Input: part model. Units: mm. Frame: model coordinates. Face numbers are marked on the shaded views. A direction names the side the tool comes from. Coordinates: 2 decimals unless noted, no trailing zeros. Order: outer loops, then holes, each group sorted by start corner. A loop starts at its lowest first (then second) coordinate and runs counter-clockwise, first axis right, second up. Notation, with made-up numbers: (-12, 88.25) - (3, 88.25) arc R26 cw to (3, 124.25) - close; hole circle Ø6 at (46.5, -21.5). An arc over 180 degrees is marked (long way). Use a Markdown table: item, result. Add a question column.
from build123d import *

# Parameters (mm, degrees)
SKETCH_1_W               = 13
SKETCH_1_H               = 10
SKETCH_1_R               = 1.2
EXTRUDE_1_DEPTH          = 6
EXTRUDE_2_DEPTH          = 24
EXTRUDE_7_DEPTH          = 20
CUT_EXTRUDE_1_DEPTH      = 33.837810475
CUT_EXTRUDE_1_DEPTH_BACK = 33.837810475
SKETCH_5_R               = 0.975
SKETCH_6_R               = 0.975
CUT_EXTRUDE_2_DEPTH      = 34.519722504
SWEEP_1_ANGLE            = 90


# Read off the part's stored shape, not the designer's step: ｽｲｰﾌﾟ1
with BuildPart() as part:
    # ｽｹｯﾁ1 → ﾎﾞｽ - 押し出し1 (new body)
    with BuildSketch(Plane(origin=(0, 0, 0), x_dir=(1, 0, 0), z_dir=(0, 1, 0))):
        Rectangle(SKETCH_1_W, SKETCH_1_H)
        with Locations(Location((0, 0, 0), (0, 0, 270))):
            Circle(SKETCH_1_R, mode=Mode.SUBTRACT)
    extrude(amount=EXTRUDE_1_DEPTH)

    # ｽｹｯﾁ2 → ﾎﾞｽ - 押し出し2 (add)
    with BuildSketch(Plane.XY.offset(5)):
        Polygon((-6.5, 6), (-8.5, 6), (-12.5, -0.92820323), (-12.5, -6.42820323), (-6.5, -6.42820323), align=None)
    extrude(amount=-EXTRUDE_2_DEPTH)

    # ｽｹｯﾁ4 → ﾎﾞｽ - 押し出し7 (add)
    with BuildSketch(Plane(origin=(-6.5, 0, 0), x_dir=(0, 0, -1), z_dir=(1, 0, 0))):
        Polygon((-5, 6), (-7, 6), (-11, -0.92820323), (-11, -6.42820323), (-7, -6.42820323), (-7, 0), (-5, 0), align=None)
    extrude(amount=EXTRUDE_7_DEPTH)

    # ｽｹｯﾁ5 → ｶｯﾄ - 押し出し1 (cut, two sides: drawn at the far end of the back side and taken through both)
    with BuildSketch(Plane.ZY.offset(12.5).offset(-CUT_EXTRUDE_1_DEPTH_BACK)):
        with Locations((-13.15, -3.67820323)):
            Circle(SKETCH_5_R)
    extrude(amount=CUT_EXTRUDE_1_DEPTH + CUT_EXTRUDE_1_DEPTH_BACK, mode=Mode.SUBTRACT)

    # ｽｹｯﾁ6 → ｶｯﾄ - 押し出し2 (cut, through all)
    with BuildSketch(Plane.XY.offset(11)):
        with Locations((10, -3.67820323)):
            Circle(SKETCH_6_R)
    extrude(amount=-CUT_EXTRUDE_2_DEPTH, mode=Mode.SUBTRACT)

    # ｽｲｰﾌﾟ1 outline → ｽｲｰﾌﾟ1 (revolve)
    with BuildSketch(Plane(origin=(-6.5, 0, 5), x_dir=(-1, 0, 0), z_dir=(0, 0, -1))):
        Polygon((0, 8), (0, -6.42820323), (8, -6.42820323), (8, -0.92820323), (4, 6), (4, 8), align=None)
    revolve(axis=Axis((-6.5, 0, 5), (0, 1, 0)), revolution_arc=SWEEP_1_ANGLE)


solid = part.part
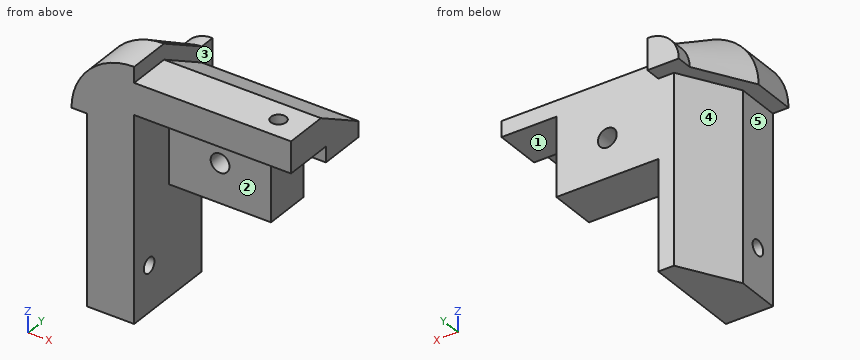
1) Material intervals for L1, parallel to X at y = -4.25, z = -9; L2, parallel to X at y = -4.5, z = 10.5; L3, parallel to Z at x = 0, y = -2.5, sorted ascending.
2) Cut plane B-B (z = 0). Return the cut outline in (x, y).
3) Cut plane D-D (y = 4.5). Return the cut outline in (x, z).
4) Cut plane C-C (y = -2). Return the cut outline in (x, z), and give its area (3 significant figures).
5) Cut plane A-A (x = 0). Return the cut outline in (y, z).
6) Reachability of the marked faces 1, 2, 3, 4 and 5 from +Z, -Z, +X, -X, +Y, -Y: full face, straight path, thin tool, end or side. Return the list, or none.
7) Contact query for flat-ended pins moving along their axis: P1, Ø3, axis at x = 4.5, y = -4, coming from the +Z side; P2, Ø1.9, axis at x = -0.5, y = -2.5, coming from the -Z side; P3, Ø1.8, axis at x = 10.5, y = 3.5, coming from the -Z side. Output: stop coordinate, or through.
Computed:
| question | item | result |
|---|---|---|
| 1 | L1 | x = -12.5 to -6.5 |
| 1 | L2 | x = -12.31 to 9.48, 10.52 to 13.5 |
| 1 | L3 | z = 7 to 11 |
| 2 | outline | (-12.5, -6.43) - (-6.5, -6.43) - (-6.5, 0) - (-1.2, 0) - (-1.2, 6) - (-8.5, 6) - (-12.5, -0.93) - close; (1.2, 0) - (6.5, 0) - (6.5, 6) - (1.2, 6) - close |
| 3 | outline | (-11.37, 5) - (-9.37, 5) - (-9.37, -19) - (-6.5, -19) - (-6.5, -5) - (6.5, -5) - (6.5, 5) - (13.5, 5) - (13.5, 7.87) - (-6.5, 7.87) - (-6.5, 9.87) arc R4.87 ccw to start; hole circle Ø2.4 at (0, 0) |
| 4 | outline | (-14.5, 5) - (-12.5, 5) - (-12.5, -19) - (-6.5, -19) - (-6.5, 7) - (13.5, 7) - (13.5, 11) - (-6.5, 11) - (-6.5, 13) arc R8 ccw to start |
| 4 | area | 274 mm2 |
| 5 | outline | (-6.43, 7) - (0, 7) - (0, 1.2) - (6, 1.2) - (6, 7) - (-0.93, 11) - (-6.43, 11) - close; (0, -5) - (6, -5) - (6, -1.2) - (0, -1.2) - close |
| 6 | face 1 | -Z, +X, +Y, -Y |
| 6 | face 2 | -Z, +X, -Y |
| 6 | face 3 | +Z, +X, +Y |
| 6 | face 4 | -Z, -X, +Y |
| 6 | face 5 | -Z, -X, +Y, -Y |
| 7 | P1 | stops at z = 11 |
| 7 | P2 | stops at z = 7 |
| 7 | P3 | stops at z = 5 |
